```python
from build123d import *

# Parameters (mm, degrees)
SKETCH1_W           = 116
SKETCH1_H           = 34.5
BOSS_EXTRUDE1_DEPTH = 3.175
SKETCH2_R           = 2
SKETCH2_R_2         = 1.25
CUT_EXTRUDE1_DEPTH  = 95.79098388
SKETCH3_W           = 116
SKETCH3_H           = 3.175
BOSS_EXTRUDE2_DEPTH = 14.1986
SKETCH4_W           = 116
SKETCH4_H           = 3.175
BOSS_EXTRUDE3_DEPTH = 26.9748
SKETCH6_R           = 3.678354521
SKETCH6_R_2         = 3.671158805
BOSS_EXTRUDE4_DEPTH = 6.35
SKETCH7_W           = 14.431210835
SKETCH7_H           = 30.1498
CUT_EXTRUDE2_DEPTH  = 6.35


with BuildPart() as part:
    # Sketch1 → Boss-Extrude1 (new body)
    with BuildSketch(Plane.XY):
        with Locations((-29, -20.25)):
            Rectangle(SKETCH1_W, SKETCH1_H)
    extrude(amount=BOSS_EXTRUDE1_DEPTH)

    # Sketch2 → Cut-Extrude1 (cut, through all)
    with BuildSketch(Plane(origin=(0, 0, 0), x_dir=(-1, 0, 0), z_dir=(0, 0, -1))):
        with Locations((-24.25, -22.13)):
            Circle(SKETCH2_R)
        with Locations((-24.25, -12.13)):
            Circle(SKETCH2_R)
        with Locations((24.25, -12.13)):
            Circle(SKETCH2_R)
        with Locations((24.25, -22.13)):
            Circle(SKETCH2_R)
        with Locations((33.75, -12.13)):
            Circle(SKETCH2_R)
        with Locations((33.75, -22.13)):
            Circle(SKETCH2_R)
        with Locations((82.25, -12.13)):
            Circle(SKETCH2_R)
        with Locations((82.25, -22.13)):
            Circle(SKETCH2_R)
        with Locations((72.699747468, -30.449747468)):
            Circle(SKETCH2_R_2)
        with Locations((65, -12.13)):
            Circle(SKETCH2_R_2)
        with Locations((51, -12.13)):
            Circle(SKETCH2_R_2)
        with Locations((43.300252532, -30.449747468)):
            Circle(SKETCH2_R_2)
        with Locations((14.699747468, -30.449747468)):
            Circle(SKETCH2_R_2)
        with Locations((7, -12.13)):
            Circle(SKETCH2_R_2)
        with Locations((-7, -12.13)):
            Circle(SKETCH2_R_2)
        with Locations((-14.699747468, -30.449747468)):
            Circle(SKETCH2_R_2)
    extrude(amount=-CUT_EXTRUDE1_DEPTH, mode=Mode.SUBTRACT)

    # Sketch3 → Boss-Extrude2 (add)
    with BuildSketch(Plane(origin=(0, -3, 0), x_dir=(1, 0, 0), z_dir=(0, 1, 0))):
        with Locations((-29, -1.5875)):
            Rectangle(SKETCH3_W, SKETCH3_H)
    extrude(amount=BOSS_EXTRUDE2_DEPTH)

    # Sketch4 → Boss-Extrude3 (add)
    with BuildSketch(Plane(origin=(0, 0, 0), x_dir=(-1, 0, 0), z_dir=(0, 0, -1))):
        with Locations((29, 9.6111)):
            Rectangle(SKETCH4_W, SKETCH4_H)
    extrude(amount=BOSS_EXTRUDE3_DEPTH)

    # Sketch6 → Boss-Extrude4 (add)
    with BuildSketch(Plane.XZ.offset(-8.0236)):
        with Locations(Location((10.05, -14.77, 0), (0, 0, 90))):
            Circle(SKETCH6_R)
        with Locations(Location((-68.05, -14.97, 0), (0, 0, 90))):
            Circle(SKETCH6_R_2)
    extrude(amount=BOSS_EXTRUDE4_DEPTH)

    # Sketch7 → Cut-Extrude2 (cut)
    with BuildSketch(Plane(origin=(0, 11.1986, 0), x_dir=(1, 0, 0), z_dir=(0, 1, 0))):
        with Locations((-79.784394582, 11.8999)):
            Rectangle(SKETCH7_W, SKETCH7_H)
        with Locations((21.784394583, 11.8999)):
            Rectangle(SKETCH7_W, SKETCH7_H)
    extrude(amount=-CUT_EXTRUDE2_DEPTH, mode=Mode.SUBTRACT)


solid = part.part
```
Read the model definition and answer for the solid it produces. Units are mm, in the model's axes. A direction names the side the tool comes from. Coordinates: 2 decimals unless noted, no trailing zeros. Order: outer loops, then holes, each group sorted by start corner. A loop starts at its lowest first (then second) coordinate and runs counter-clockwise, first axis right, second up. Notation, with made-up numbers: (37.25, -21.5) - (93.25, -21.5) arc R33 ccw to (93.25, 9.5) - close; hole circle Ø9 at (-15.5, 46.25). An arc over 180 degrees is marked (long way). Answer as a JSON object with one key per item and string values. Group by question number.
Item 1: Section D-D (z = -14.97) is taken. Give the vertices of the cut face in (x, y), plus the area to 3 significant figures.
Item 2: Section C-C (y = 3) is taken. Give the vertices of the cut face in (x, z) (3 decimals).
Item 3: A tool of negligible diameter and unlimited length cuts with its end or side. For faces 4 (the face through (14.569, 9, -12)), 5 (the face through (-30, -37.5, 2)), from which of +Z, -Z, +X, -X, +Y, -Y can it reach the whole face along a straight path? Write none if from no direction.
Item 4: Section B-B (x = -51) is taken. Give the vertices of the cut face in (y, z) (3 decimals).
Item 5: Section A-A (x = 24.25) is taken. Give the vertices of the cut face in (y, z) (3 decimals).
Item 6: The mould has two halves that part along Y. Classify faces 1 (the face through (-66.19, -11.75, 1.57)), 2 (the face through (-28, 11.199, -12)), 3 (the face through (-30, -15, 0)): +Y half, -Y half, draft (parallel to the pull), parting line (faces both ways), or undercut.
Item 7: Consider probe 1 along Y at (x, z) = (24, 1); probe 2 along Y at (x, z) = (-65, 1); probe 3 along Z at (x, y) = (23, -16.5) (3 decimals). Determine where each line is inside the solid, lowest interval first. Write a range as from..to.
Item 8: Flat-ended cylindrical pins translate along their axes: P1, Ø10, axis at x = -73, y = -12.5, coming from the -Z side; P2, Ø8, axis at x = -30.5, z = -10.5, coming from the -Y side; P3, Ø3, axis at x = -65, y = -12.13, coming from the +Z side (3 decimals); P4, Ø5, axis at y = 7.5, z = -10, coming from the +X side. Find the tip coordinate at first contact, or state that the pin passes through.
Results are:
{
 "1": {"outline": "(-72.57, 8.02) - (-71.72, 8.02) - (-71.72, 1.67) - (-64.38, 1.67) - (-64.38, 8.02) - (6.38, 8.02) - (6.38, 1.67) - (13.72, 1.67) - (13.72, 8.02) - (14.57, 8.02) - (14.57, 11.2) - (-72.57, 11.2) - close", "area": "370 mm^2"},
 "2": {"outline": "(-87, 0) - (29, 0) - (29, 3.175) - (-87, 3.175) - close; circle Ø7.342 at (-68.05, -14.97); circle Ø7.357 at (10.05, -14.77)"},
 "3": {"face 4": "+Z, -Z, +X, +Y", "face 5": "+Z, -Z, +X, -X, -Y"},
 "4": {"outline": "(-37.5, 0) - (-13.38, 0) - (-13.38, 3.175) - (-37.5, 3.175) - close; (-10.88, 0) - (8.024, 0) - (8.024, -26.975) - (11.199, -26.975) - (11.199, 3.175) - (-10.88, 3.175) - close"},
 "5": {"outline": "(-37.5, 0) - (-24.13, 0) - (-24.13, 3.175) - (-37.5, 3.175) - close; (-20.13, 0) - (-14.13, 0) - (-14.13, 3.175) - (-20.13, 3.175) - close; (-10.13, 0) - (4.849, 0) - (4.849, 3.175) - (-10.13, 3.175) - close"},
 "6": {"face 1": "undercut", "face 2": "+Y half", "face 3": "draft"},
 "7": {"probe 1": "y = -37.5..-24.11, -20.15..-14.11, -10.15..4.85", "probe 2": "y = -37.5..-13.38, -10.88..11.2", "probe 3": "z = 0..3.175"},
 "8": {"P1": "stops at z = 0", "P2": "stops at y = 8.02", "P3": "stops at z = 3.175", "P4": "stops at x = 14.57"}
}
